from build123d import *

# Parameters (mm, degrees)
EXTRUDE_1_DEPTH = 130


with BuildPart() as part:
    # 草图1 → 凸台-拉伸1 (new, symmetric)
    with BuildSketch(Plane(origin=(0, 0, 0), x_dir=(0, 0, -1), z_dir=(1, 0, 0))):
        with BuildLine():
            Line((17.5, 0), (14.94151844, 0))
            ThreePointArc((14.94151844, 0), (13.772097871, 0.37751563), (13.044151844, 1.367544468))
            Line((13.044151844, 1.367544468), (11.955848156, 4.632455532))
            ThreePointArc((11.955848156, 4.632455532), (11.227902129, 5.62248437), (10.05848156, 6))
            Line((10.05848156, 6), (-10.05848156, 6))
            ThreePointArc((-10.05848156, 6), (-11.227902129, 5.62248437), (-11.955848156, 4.632455532))
            Line((-11.955848156, 4.632455532), (-13.044151844, 1.367544468))
            ThreePointArc((-13.044151844, 1.367544468), (-13.772097871, 0.37751563), (-14.94151844, 0))
            Line((-14.94151844, 0), (-17.5, 0))
            Line((-17.5, 0), (-17.5, 1.2))
            Line((-17.5, 1.2), (-14.94151844, 1.2))
            ThreePointArc((-14.94151844, 1.2), (-14.473750212, 1.351006252), (-14.182571802, 1.747017787))
            Line((-14.182571802, 1.747017787), (-13.094268114, 5.011928851))
            ThreePointArc((-13.094268114, 5.011928851), (-11.929554471, 6.595974993), (-10.05848156, 7.2))
            Line((-10.05848156, 7.2), (10.05848156, 7.2))
            ThreePointArc((10.05848156, 7.2), (11.929554471, 6.595974993), (13.094268114, 5.011928851))
            Line((13.094268114, 5.011928851), (14.182571802, 1.747017787))
            ThreePointArc((14.182571802, 1.747017787), (14.473750212, 1.351006252), (14.94151844, 1.2))
            Line((14.94151844, 1.2), (17.5, 1.2))
            Line((17.5, 1.2), (17.5, 0))
        make_face()
    extrude(amount=EXTRUDE_1_DEPTH, both=True)


solid = part.part
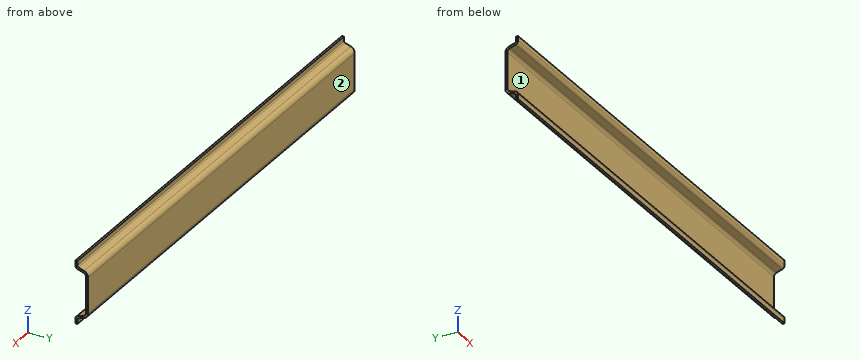
The listing builds one solid part. Answer for the finished solid, in the listing's coordinates (mm). Face numbers are marked on the shaded views. Round coordinates to 2 decimals unless told otherwise and drop trailing zeros. Order: outer loops, then holes, each group sorted by start corner. A loop starts at its lowest first (then second) coordinate and runs counter-clockwise, first axis right, second up. Notation, with made-up numbers: M 18,4.25 L 64,4.25 A16 ccw 64,25.25 Z; hole C 15,-18.5 d3. An arc over 180 degrees is marked long. Answer in a Markdown table with one row per item. Add a question column.
1) Determine the mould class of the marked faces 1 and 2 for opening direction Z: pulls with the +Z half, pulls with the -Z half, needs draft (parallel to the pull), parting line crosses it, or undercut.
2) The part is cut by section A-A on x = 40. Determine the outline of the cut face in (y, z), plus the area to 3 significant figures.
3) Consider line 1 along Y through (x, z) = (-77, 1); line 2 along Z through (x, y) = (58.5, 1); line 3 along Z through (x, y) = (-4, 5.5). Determine where each line is inside the solid, lowest interval first. Write a range as from..to.
4) Flat-ended cylindrical pins translate along their axes: pin 1 Ø1.3 at (x, z) = (55, 16) entering from +Y; pin 2 Ø6 at (x, z) = (25, -2) entering from -Y; pin 3 Ø2 at (x, z) = (-53.5, -15.5) entering from +Y. Find the tip coordinate at first contact, or state that the pin passes through.
5) The part is cut by section B-B on z = -5. Determine the outline of the cut face in (x, y), plus the area to 3 significant figures.
Findings below:
| question | item | result |
|---|---|---|
| 1 | face 1 | undercut |
| 1 | face 2 | needs draft |
| 2 | outline | M 0,-17.5 L 1.2,-17.5 L 1.2,-14.94 A0.8 cw 1.75,-14.18 L 5.01,-13.09 A3.2 ccw 7.2,-10.06 L 7.2,10.06 A3.2 ccw 5.01,13.09 L 1.75,14.18 A0.8 cw 1.2,14.94 L 1.2,17.5 L 0,17.5 L 0,14.94 A2 ccw 1.37,13.04 L 4.63,11.96 A2 cw 6,10.06 L 6,-10.06 A2 cw 4.63,-11.96 L 1.37,-13.04 A2 ccw 0,-14.94 Z |
| 2 | area | 50.5 mm² |
| 3 | line 1 | y = 6..7.2 |
| 3 | line 2 | z = -17.5..-13.21, 13.21..17.5 |
| 3 | line 3 | z = -12.89..-11.38, 11.38..12.89 |
| 4 | pin 1 | stops at y = 1.2 |
| 4 | pin 2 | stops at y = 6 |
| 4 | pin 3 | stops at y = 1.33 |
| 5 | outline | M -130,6 L 130,6 L 130,7.2 L -130,7.2 Z |
| 5 | area | 312 mm² |
